Design review of the part built by this model. Coordinates are the model's own, in mm. A direction names the side the tool comes from. Coordinates: 2 decimals unless noted, no trailing zeros. Loops run counter-clockwise (first coordinate to the right, second up) from the corner with the lowest first, then second, coordinate; pieces in that order, holes last. Notation, with made-up numbers: (37.5, 48.25) -> (48.5, 48.25) arc R31 ccw to (48.5, 80.25) -> close; hole circle Ø5 at (53, 70). An arc over 180 degrees is marked (long way). Answer in a Markdown table with one row per item.
```python
from build123d import *

# Parameters (mm, degrees)
F0_W     = 2.5
F0_H     = 27.965406
F1_DEPTH = 41
F2_W     = 3.093319
F2_H     = 4.968024
F2_R     = 2.421667
F3_DEPTH = 1
F4_W     = 3
F4_H     = 6
F5_DEPTH = 1
F6_W     = 39
F6_H     = 25
F7_DEPTH = 0.5


with BuildPart() as f1:
    # F0 (on Right) → F1 (new body)
    with BuildSketch(Plane.YZ):
        with BuildLine():
            Line((-13.671529, 14.816766), (-18.471529, 14.816766))
            ThreePointArc((-18.471529, 14.816766), (-21.299956, 13.645193), (-22.471529, 10.816766))
            Line((-22.471529, 10.816766), (-22.471529, -18.683234))
            ThreePointArc((-22.471529, -18.683234), (-21.299956, -21.511661), (-18.471529, -22.683234))
            Line((-18.471529, -22.683234), (-16.671529, -22.683234))
            ThreePointArc((-16.671529, -22.683234), (-14.550208, -21.804554), (-13.671529, -19.683234))
            Line((-13.671529, -19.683234), (-13.671529, 5.316766))
            Line((-13.671529, 5.316766), (-13.671529, 9.816766))
            Line((-13.671529, 9.816766), (-13.671529, 14.816766))
        make_face()
        Polygon((-8.671529, 9.816766), (-13.671529, 9.816766), (-13.671529, 5.316766), (-11.171529, 5.316766), (-8.671529, 5.316766), align=None)
        Polygon((-8.671529, 9.816766), (-13.671529, 14.816766), (-13.671529, 9.816766), align=None)
        with Locations((-9.921529, -8.665937)):
            Rectangle(F0_W, F0_H)
    extrude(amount=F1_DEPTH)

    # F2 (on face) → F3 (join)
    with BuildSketch(Plane.YZ.offset(41)):
        with Locations((-18.047974, 2.484012)):
            Rectangle(F2_W, F2_H)
        with Locations((-18.139437, -5.160558)):
            Circle(F2_R)
    extrude(amount=F3_DEPTH)

    # F4 (on face) → F5 (join)
    with BuildSketch(Plane(origin=(0, 0, 0), x_dir=(0, -1, 0), z_dir=(-1, 0, 0))):
        with Locations((18.208981, 2.310598)):
            Rectangle(F4_W, F4_H)
        with Locations((18.208981, -7.405368)):
            Rectangle(F4_W, F4_H)
    extrude(amount=F5_DEPTH)

    # F6 (on face) → F7 (cut)
    with BuildSketch(Plane.XZ.offset(22.471529)):
        with Locations((20.5, -2.683234)):
            Rectangle(F6_W, F6_H)
    extrude(amount=-F7_DEPTH, mode=Mode.SUBTRACT)


solid = f1.part
```
(1) To check wall thickness, follow probe 1 along Y at (x, z) = (16.5, -6); probe 2 along Y at (x, z) = (31.5, -18); probe 3 along X at (y, z) = (-15, 8). State the ranges of each line that lie inside material, in increasing order.
Evaluation:
| item | result |
|---|---|
| probe 1 | y = -21.97 to -13.67, -11.17 to -8.67 |
| probe 2 | y = -22.47 to -13.67, -11.17 to -8.67 |
| probe 3 | x = 0 to 41 |
(2) Take a section at B-B on x = 6. Give the boundary of the cut face in (y, z), and give its area (3 significant figures).
Evaluation:
| item | result |
|---|---|
| outline | (-22.47, -18.68) arc R4 ccw to (-18.47, -22.68) -> (-16.67, -22.68) arc R3 ccw to (-13.67, -19.68) -> (-13.67, 5.32) -> (-11.17, 5.32) -> (-11.17, -22.65) -> (-8.67, -22.65) -> (-8.67, 9.82) -> (-13.67, 14.82) -> (-18.47, 14.82) arc R4 ccw to (-22.47, 10.82) -> (-22.47, 9.82) -> (-21.97, 9.82) -> (-21.97, -15.18) -> (-22.47, -15.18) -> close |
| area | 414 mm² |
(3) For pin 1 (0.8 mm diameter, centred on x = 41.5, z = 1.5, fed in from -Y); pin 2 (8.5 mm diameter, centred on x = 24, z = -8, fed in from -Y); pin 3 (8 mm diameter, centred on x = 14, y = -11.5, fed in from -Z); pin 4 (1.1 mm diameter, centred on x = -0.5, z = 1.5, fed in from +Y), all flat-tipped, find the tip position at first contact; note any pin that passes through.
Evaluation:
| item | result |
|---|---|
| pin 1 | stops at y = -19.59 |
| pin 2 | stops at y = -21.97 |
| pin 3 | stops at z = -22.65 |
| pin 4 | stops at y = -8.67 |
(4) Take a section at D-D on z = -17.5. Give the boundary of the cut face in (x, y), and give its area (3 significant figures).
Evaluation:
| item | result |
|---|---|
| outline | (0, -22.47) -> (41, -22.47) -> (41, -13.67) -> (0, -13.67) -> close; (0, -11.17) -> (41, -11.17) -> (41, -8.67) -> (0, -8.67) -> close |
| area | 463 mm² |
(5) Take a section at C-C on y = -18. Give the boundary of the cut face in (x, z), and give its area (3 significant figures).
Evaluation:
| item | result |
|---|---|
| outline | (-1, -10.41) -> (0, -10.41) -> (0, -22.68) -> (41, -22.68) -> (41, -7.58) -> (42, -7.58) -> (42, -2.74) -> (41, -2.74) -> (41, 0) -> (42, 0) -> (42, 4.97) -> (41, 4.97) -> (41, 14.82) -> (0, 14.82) -> (0, 5.31) -> (-1, 5.31) -> (-1, -0.69) -> (0, -0.69) -> (0, -4.41) -> (-1, -4.41) -> close |
| area | 1,560 mm² |
(6) Draft analysis for pull direction Z (two halves, no side actions). For faces 5 (the flat face through (41.5, -18.1, 0)), 6 (the flat face through (-0.5, -18.2, 5.311)), 7 (the flat face through (-1, -18, -7)), 8 (the flat face through (20, -18, -22.683)), state which applies: pulls with the +Z half, pulls with the -Z half, needs draft (parallel to the pull), parting line crosses it, or undercut.
Evaluation:
| item | result |
|---|---|
| face 5 | undercut |
| face 6 | pulls with the +Z half |
| face 7 | needs draft |
| face 8 | pulls with the -Z half |
(7) Take a section at A-A on z = 0.5. Give the boundary of the cut face in (x, y).
Evaluation:
| item | result |
|---|---|
| outline | (-1, -19.71) -> (0, -19.71) -> (0, -22.47) -> (1, -22.47) -> (1, -21.97) -> (40, -21.97) -> (40, -22.47) -> (41, -22.47) -> (41, -19.59) -> (42, -19.59) -> (42, -16.5) -> (41, -16.5) -> (41, -13.67) -> (0, -13.67) -> (0, -16.71) -> (-1, -16.71) -> close; (0, -11.17) -> (41, -11.17) -> (41, -8.67) -> (0, -8.67) -> close |
(8) Tool access review of faces 1 (the cylindrical face through (41.49, -20.56, -5.05)), 2 (the flat face through (-0.5, -18.2, -0.689)), 3 (the flat face through (-0.5, -19.709, -7.4)), 4 (the flat face through (20, -12, 5.317)): name each direction out of +Z, -Z, +X, -X, +Y, -Y from which nothing blocks a thin tool from reaching the whole face with its end or side.
Evaluation:
| item | result |
|---|---|
| face 1 | +X |
| face 2 | -X, +Y, -Y |
| face 3 | +Z, -Z, -X, -Y |
| face 4 | -Z, +X, -X |
